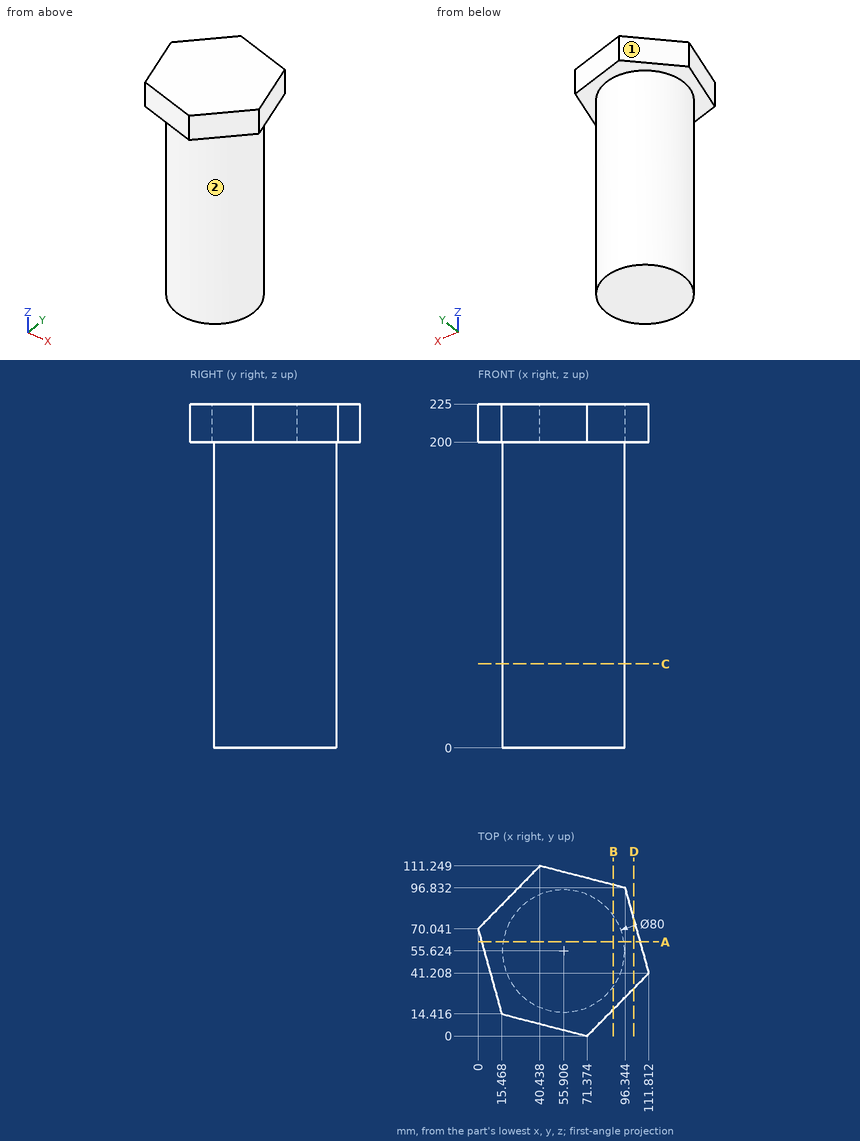
For this review, use the dimensioned drawing (mm, ordinates from the lowest corner) and the shaded views. A direction names the side the tool comes from. Give positions to 0.01 mm unless a question says otherwise; leave off trailing zeros. Order: outer loops, then holes, each group sorted by start corner. A loop starts at its lowest first (then second) coordinate and runs counter-clockwise, first axis right, second up. Notation, with made-up numbers: (-17.5, 31.25) - (-12.5, 31.25) arc R27 ccw to (-12.5, 47.25) - close; hole circle Ø11 at (18, 17). An arc over 180 degrees is marked (long way). Use CSV: the item, a comma, the result in double quotes. Start each with the question number.
Q1. Tool access review of the marked faces 1 and 2: name each direction out of +Z, -Z, +X, -X, +Y, -Y from which nothing blocks a thin tool from reaching the whole face with its end or side.
Q2. We need section B-B, the plane x = 88.5. Write out the cut boundary in (y, z) (1 decimal).
Q3. Clearance check with flat-ended pins moving along their axes: pin 1 Ø2 at (y, z) = (90, 46.5) entering from +X (1 decimal); pin 2 Ø2 at (x, z) = (81, 59) entering from -Y (1 decimal); pin 3 Ø3 at (y, z) = (72.5, 148.5) entering from +X. State where each tip first meets the part, or that it passes through.
Q4. To check wall thickness, follow line 1 along Z through (x, y) = (104, 57.5); line 2 along Y through (x, z) = (67.5, 184.5); line 3 along X through (y, z) = (72.5, 199). State the ranges of each line that lie inside material, in increasing order. Write a range as [from, to].
Q5. We need section A-A, the plane y = 61.5. Write out the cut boundary in (x, z) (1 decimal), and give its area (3 significant figures).
Q6. We need section C-C, the plane z = 55. Write out the cut boundary in (x, y) (1 decimal), and give its area (3 significant figures).
Q7. We need section D-D, the plane x = 102. Write out the cut boundary in (y, z).
Outcome:
1,face 1,"+Z, -Z, -X, +Y"
1,face 2,"-Z"
2,outline,"(17.5, 200) - (32.4, 200) - (32.4, 0) - (78.8, 0) - (78.8, 200) - (98.9, 200) - (98.9, 225) - (17.5, 225) - close"
3,pin 1,"stops at x = 78"
3,pin 2,"stops at y = 23.7"
3,pin 3,"stops at x = 92.83"
4,line 1,"z = [200, 225]"
4,line 2,"y = [17.34, 93.91]"
4,line 3,"x = [19.64, 92.17]"
5,outline,"(2.4, 200) - (16.3, 200) - (16.3, 0) - (95.5, 0) - (95.5, 200) - (106.2, 200) - (106.2, 225) - (2.4, 225) - close"
5,area,"18,400 mm^2"
6,outline,"circle Ø80 at (55.9, 55.6)"
6,area,"5,030 mm^2"
7,outline,"(31.21, 200) - (76.49, 200) - (76.49, 225) - (31.21, 225) - close"
